from build123d import *

# Parameters (mm, degrees)
SKETCH1_W                               = 160
SKETCH1_H                               = 45
BOSS_EXTRUDE1_DEPTH                     = 12
CBORE_FOR_M5_HEX_HEAD_BOLT5_D           = 4.5
CBORE_FOR_M5_HEX_HEAD_BOLT5_CBORE_D     = 10
CBORE_FOR_M5_HEX_HEAD_BOLT5_CBORE_DEPTH = 5
CBORE_FOR_M5_HEX_HEAD_BOLT7_D           = 4.5
CBORE_FOR_M5_HEX_HEAD_BOLT7_CBORE_D     = 10
CBORE_FOR_M5_HEX_HEAD_BOLT7_CBORE_DEPTH = 5
CUT_EXTRUDE4_DEPTH                      = 12


with BuildPart() as part:
    # Sketch1 → Boss-Extrude1 (new body)
    with BuildSketch(Plane(origin=(0, 0, 0), x_dir=(1, 0, 0), z_dir=(0, 1, 0))):
        with Locations((-80, -22.5)):
            Rectangle(SKETCH1_W, SKETCH1_H)
    extrude(amount=BOSS_EXTRUDE1_DEPTH)

    # CBORE for M5 Hex Head Bolt5 (through all)
    with Locations(Plane(origin=(0, 0, 0), x_dir=(-1, 0, 0), z_dir=(0, -1, 0))):
        with Locations((152.334853244, -7.222273521)):
            CounterBoreHole(CBORE_FOR_M5_HEX_HEAD_BOLT5_D / 2, CBORE_FOR_M5_HEX_HEAD_BOLT5_CBORE_D / 2, CBORE_FOR_M5_HEX_HEAD_BOLT5_CBORE_DEPTH)

    # CBORE for M5 Hex Head Bolt7 (through all)
    with Locations(Plane(origin=(0, 0, 0), x_dir=(-1, 0, 0), z_dir=(0, -1, 0))):
        with Locations((7.319954145, -7.319990423)):
            CounterBoreHole(CBORE_FOR_M5_HEX_HEAD_BOLT7_D / 2, CBORE_FOR_M5_HEX_HEAD_BOLT7_CBORE_D / 2, CBORE_FOR_M5_HEX_HEAD_BOLT7_CBORE_DEPTH)

    # Sketch17 → Cut-Extrude4 (cut)
    with BuildSketch(Plane(origin=(0, 0, 0), x_dir=(-1, 0, 0), z_dir=(0, -1, 0))):
        with BuildLine():
            ThreePointArc((145, -35), (150, -30), (145, -25))
            Line((145, -25), (15, -25))
            ThreePointArc((15, -25), (10, -30), (15, -35))
            Line((15, -35), (145, -35))
        make_face()
    extrude(amount=-CUT_EXTRUDE4_DEPTH, mode=Mode.SUBTRACT)


solid = part.part
The listing builds one solid part. Answer for the finished solid, in the listing's coordinates (mm). A direction names the side the tool comes from. Round coordinates to 2 decimals unless told otherwise and drop trailing zeros. Order: outer loops, then holes, each group sorted by start corner. A loop starts at its lowest first (then second) coordinate and runs counter-clockwise, first axis right, second up. Notation, with made-up numbers: (73, -21) -> (87, -21) arc R30 cw to (87, 12) -> close; hole circle Ø8 at (69.5, 2.5). An arc over 180 degrees is marked (long way). One line per item, written item: value.
Item 1: Given P1, Ø5, axis at x = -7.32, z = 7.32, coming from the -Y side, flat-ended and moving along its own axis, determine where the tip first touches the part or whether it passes through.
Taken from the geometry:
P1: stops at y = 5
Item 2: For a pull along X with two mould halves and no side action, classify faces 4 (the flat face through (-81, 6, 45)), 5 (the flat face through (-9.5, 5, 8.4)), 6 (the flat face through (0, 6, 23)), 7 (the cylindrical face through (-3.35, 2.46, 10.36)) as released by +X, released by -X, zero draft, split by the parting line, or undercut.
Taken from the geometry:
face 4: zero draft
face 5: undercut
face 6: released by +X
face 7: undercut
Item 3: For faces 1 (the flat face through (-154.5, 5, 8.3)), 2 (the flat face through (-81, 6, 0)), 3 (the flat face through (-81, 6, 25)), determine the directions among +Z, -Z, +X, -X, +Y, -Y from which every point of the face is accessible in a straight line to the end or side of a thin tool.
Taken from the geometry:
face 1: -Y
face 2: -Z, +X, -X, +Y, -Y
face 3: +Y, -Y
Item 4: Find section A-A, the plane x = -126.5. Give the vertices of the cut face in (y, z).
Taken from the geometry:
outline: (0, 0) -> (12, 0) -> (12, 25) -> (0, 25) -> close; (0, 35) -> (12, 35) -> (12, 45) -> (0, 45) -> close
Item 5: Find section B-B, the plane z = 27.5. Give the vertices of the cut face in (x, y), then the cut area to 3 significant figures.
Taken from the geometry:
outline: (-160, 0) -> (-149.33, 0) -> (-149.33, 12) -> (-160, 12) -> close; (-10.67, 0) -> (0, 0) -> (0, 12) -> (-10.67, 12) -> close
area: 256 mm2
Item 6: Find section C-C, the plane y = 2. Give the vertices of the cut face in (x, z), then the cut area to 3 significant figures.
Taken from the geometry:
outline: (-160, 0) -> (0, 0) -> (0, 45) -> (-160, 45) -> close; hole circle Ø10 at (-152.33, 7.22); hole (-145, 25) -> (-15, 25) arc R5 ccw to (-15, 35) -> (-145, 35) arc R5 ccw to start; hole circle Ø10 at (-7.32, 7.32)
area: 5,660 mm2
Item 7: Straight lines are drawn through the part: L1, parallel to X at y = 4.5, z = 7; L2, parallel to Z at x = -106, y = 1.5; L3, parallel to Y at x = -9.5, z = 6. For each, find the intervals that lie inside material, in ascending order.
Taken from the geometry:
L1: x = -160 to -157.33, -147.34 to -12.31, -2.33 to 0
L2: z = 0 to 25, 35 to 45
L3: y = 5 to 12
